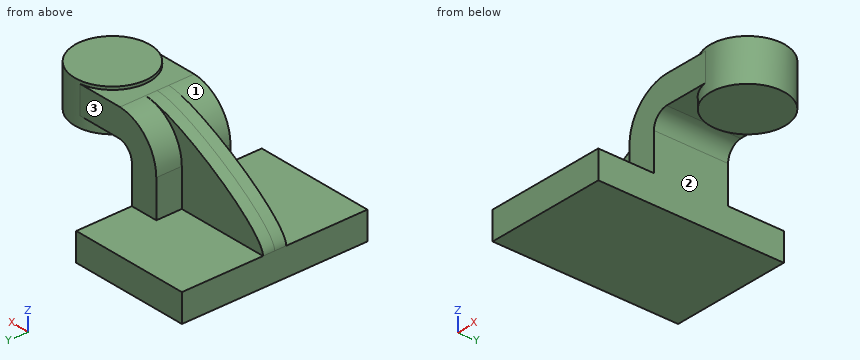
```python
from build123d import *

# Parameters (mm, degrees)
F1_DEPTH = 63.5
F0_W     = 25.1334723711
F0_H     = 19.05
F2_DEPTH = 25.4
F3_DEPTH = 7.9375


with BuildPart() as f1:
    # F0 (on Front) → F1 (new body, symmetric)
    with BuildSketch(Plane.XZ):
        Polygon((-41.275, 9.525), (-41.275, -9.525), (41.275, -9.525), (41.275, 9.525), (22.225, 9.525), align=None)
    extrude(amount=F1_DEPTH, both=True)

    # F0 (on Front) → F2 (join, symmetric)
    with BuildSketch(Plane.XZ):
        with BuildLine():
            Line((22.225, 9.525), (41.275, 9.525))
            Line((41.275, 9.525), (41.275, 35.0430520255))
            ThreePointArc((41.275, 35.0430520255), (44.1109864464, 42.2590514087), (51.101194276, 45.6132220545))
            Line((51.101194276, 45.6132220545), (60.325, 45.6132220545))
            Line((60.325, 45.6132220545), (60.325, 64.6632220545))
            Line((60.325, 64.6632220545), (50.5813328098, 64.6632220545))
            ThreePointArc((50.5813328098, 64.6632220545), (30.4568754428, 55.5457108956), (22.225, 35.0430520255))
            Line((22.225, 35.0430520255), (22.225, 9.525))
        make_face()
        with Locations((72.8917361856, 55.1382220545)):
            Rectangle(F0_W, F0_H)
    extrude(amount=F2_DEPTH, both=True)

    # F0 (on Front) → F3 (join, symmetric)
    with BuildSketch(Plane.XZ):
        with BuildLine():
            add(Edge.make_bspline(
                [(-41.275, 9.525), (-40.6684018672, 25.3735426813), (27.1178521216, 64.2672926188), (50.5813328098, 64.6632220545)],
                knots=[0, 0, 0, 0, 107.134538822, 107.134538822, 107.134538822, 107.134538822], degree=3))
            Line((-41.275, 9.525), (22.225, 9.525))
            Line((22.225, 9.525), (22.225, 35.0430520255))
            ThreePointArc((22.225, 35.0430520255), (30.4568754428, 55.5457108956), (50.5813328098, 64.6632220545))
        make_face()
    extrude(amount=F3_DEPTH, both=True)

    # F0 (on Front) → F4 (revolve)
    with BuildSketch(Plane.XZ):
        Polygon((85.4584723711, 66.675), (85.4584723711, 64.6632220545), (85.4584723711, 45.6132220545), (85.4584723711, 38.1), (111.125, 38.1), (111.125, 66.675), align=None)
    revolve(axis=Axis((85.4584723711, 0, 52.3875), (0, 0, 1)))


solid = f1.part
```
Input: part model. Units: mm. Frame: model coordinates. Face numbers are marked on the shaded views. A direction names the side the tool comes from. Give positions to 0.01 mm unless a question says otherwise; leave off trailing zeros. Write each loop counter-clockwise with the first axis right and the second up, starting at its lowest first coordinate (ties: lowest second). Pieces come first, ordered by that corner, then holes. Notation, with made-up numbers: (-36.75, 15.25) - (-26.75, 15.25) arc R31 ccw to (-26.75, 42.25) - close; hole circle Ø11 at (-34, 12). An arc over 180 degrees is marked (long way). Write item = value, one per line. Start each with the question number.
1) Cut plane B-B (x = 65). Return loops of the section in (y, z) (3 decimals).
2) Pin query (flat end, axial travel): pin 1 (8 mm diameter, centred on x = 29.5, y = 35.5, fed in from +Z) (3 decimals); pin 2 (10 mm diameter, centred on x = 23, y = -15, fed in from +Z); pin 3 (22.5 mm diameter, centred on y = -15, z = 16.5, fed in from +X) (3 decimals); pin 4 (8 mm diameter, centred on x = -5, z = 10, fed in from +Y). Return the tip coordinate at first contact, or that it passes through.
3) Cut plane A-A (y = 49). Return loops of the section in (x, z) (3 decimals).
4) Reachability of the marked faces 1, 2 and 3 from +Z, -Z, +X, -X, +Y, -Y: full face, straight path, thin tool, end or side. Return the list, or none.
5) Material intervals for L1, parallel to Z at x = 37, y = -43 (3 decimals); L2, parallel to X at y = -22.5, z = 30 (3 decimals); L3, parallel to Y at x = 3, z = 46.5, sorted ascending. Write a range as [from, to].
Answers follow:
q1.outline = (-25.4, 45.613) - (-15.499, 45.613) - (-15.499, 38.1) - (15.499, 38.1) - (15.499, 45.613) - (25.4, 45.613) - (25.4, 64.663) - (15.499, 64.663) - (15.499, 66.675) - (-15.499, 66.675) - (-15.499, 64.663) - (-25.4, 64.663) - close
q2.pin_1 = 9.525
q2.pin_2 = 52.62
q2.pin_3 = 41.275
q2.pin_4 = 63.5
q3.outline = (-41.275, -9.525) - (41.275, -9.525) - (41.275, 9.525) - (-41.275, 9.525) - close
q4.face_1 = +Z, -X, -Y
q4.face_2 = -Z, +X, +Y, -Y
q4.face_3 = +Z, -X, +Y
q5.L1 = [-9.525, 9.525]
q5.L2 = [22.225, 41.275]
q5.L3 = [-7.94, 7.94]
